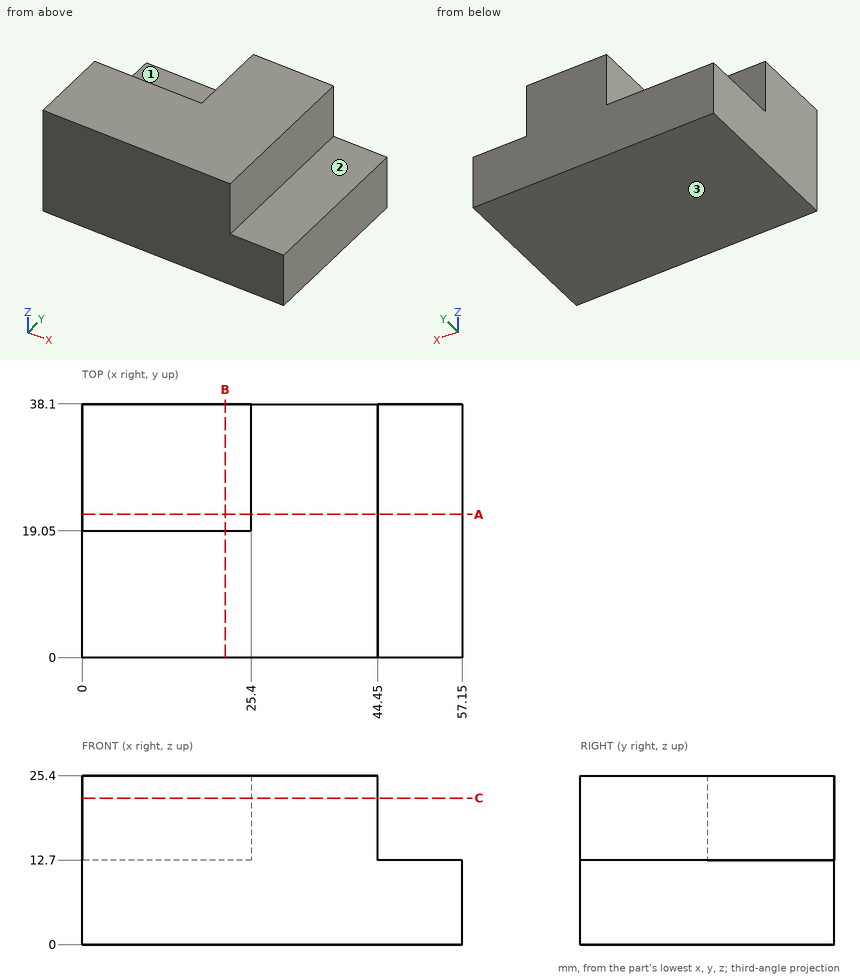
Can you work these out from the drawing? Everything is in mm from the part's minimum corner. A direction names the side the tool comes from. Coordinates: 2 decimals unless noted, no trailing zeros. Loops run counter-clockwise (first coordinate to the right, second up) from the corner with the lowest first, then second, coordinate; pieces in that order, holes last. Notation, with made-up numbers: (84, -33) - (119, -33) arc R24 ccw to (119, -22) - close; hole circle Ø5 at (71, 32). An arc over 180 degrees is marked (long way). Use a Markdown table: item, result.
Item 1: I want a section at B-B on x = 21.5. Please give me the cut outline in (y, z), and give its area (3 significant figures).
Numbers:
| item | result |
|---|---|
| outline | (0, 0) - (38.1, 0) - (38.1, 12.7) - (19.05, 12.7) - (19.05, 25.4) - (0, 25.4) - close |
| area | 726 mm2 |
Item 2: Will these pins go through, and if not, where does the flat tip stop? pin 1 (10 mm diameter, centred on y = 17.5, z = 20, fed in from +X); pin 2 (9.5 mm diameter, centred on x = 9.5, y = 31.5, fed in from +Z); pin 3 (6.5 mm diameter, centred on y = 28.5, z = 20, fed in from -X).
Numbers:
| item | result |
|---|---|
| pin 1 | stops at x = 44.45 |
| pin 2 | stops at z = 12.7 |
| pin 3 | stops at x = 25.4 |
Item 3: For the marked faces 1, 2 and 3, which set-ups out of +Z, -Z, +X, -X, +Y, -Y let a thin tool reach every point of the face, with its end or its side?
Numbers:
| item | result |
|---|---|
| face 1 | +Z, -X, +Y |
| face 2 | +Z, +X, +Y, -Y |
| face 3 | -Z, +X, -X, +Y, -Y |
Item 4: If I drill on probe 1 along X at (y, z) = (5.5, 16.75); probe 2 along Z at (x, y) = (23, 24); probe 3 along X at (y, z) = (27, 14), over which ranges is the centre line in solid material (lowest first)? Write a range as from..to.
Numbers:
| item | result |
|---|---|
| probe 1 | x = 0..44.45 |
| probe 2 | z = 0..12.7 |
| probe 3 | x = 25.4..44.45 |
Item 5: I want a section at A-A on y = 21.5. Please give me the cut outline in (x, z).
Numbers:
| item | result |
|---|---|
| outline | (0, 0) - (57.15, 0) - (57.15, 12.7) - (44.45, 12.7) - (44.45, 25.4) - (25.4, 25.4) - (25.4, 12.7) - (0, 12.7) - close |
Item 6: I want a section at C-C on z = 22. Please give me the cut outline in (x, y).
Numbers:
| item | result |
|---|---|
| outline | (0, 0) - (44.45, 0) - (44.45, 38.1) - (25.4, 38.1) - (25.4, 19.05) - (0, 19.05) - close |
